Model file for the job. Use its own axes, mm. Face numbers are marked on the shaded views. Coordinates: 2 decimals unless noted, no trailing zeros. Order: outer loops, then holes, each group sorted by start corner. A loop starts at its lowest first (then second) coordinate and runs counter-clockwise, first axis right, second up. Notation, with made-up numbers: (36.25, 69) -> (86.25, 69) arc R15 ccw to (86.25, 76) -> close; hole circle Ø4 at (54, 70.25). An arc over 180 degrees is marked (long way). Return JSON: item names as keys, results as strings. Group by question number.
1) Pull direction X, two halves, no side cores. Call the marked faces 1, 2, 3 and 4: +X half, -X half, draft (parallel to the pull), parting line (faces both ways), or undercut.
2) Flat gauge pins, fed straight in: pin 1 (1 mm diameter, centred on y = -2.5, z = 3, fed in from +X); pin 2 (1 mm diameter, centred on x = 3.5, y = 1, fed in from -Z); pin 3 (2 mm diameter, centred on x = 0.5, z = -2, fed in from +Y). Where does each tip first touch, or does it go through?
3) Cut at D-D (x = 4.75). Write the cut outline in (y, z) (1 decimal), and give its area (3 significant figures).
4) Probe line 1 (Z direction, x = -0.75, y = 0) (3 decimals); line 2 (Y direction, x = -3.75, z = 1); line 3 (Z direction, x = 4.25, y = 1). List the from-to ranges inside material, lowest first.
5) Cut at C-C (x = -4.5). Write the cut outline in (y, z) (3 decimals), and give its area (3 significant figures).
Autodesk Inventor part; units mm, degrees
ref_plane "作業平面1" through (4.5, 0, 0) normal (1, 0, 0) x (0, 0, -1)
ref_plane "YZ Plane" through (0, 0, 0) normal (1, 0, 0) x (0, 1, 0)
ref_plane "XZ Plane" through (0, 0, 0) normal (0, 1, 0) x (-1, 0, 0)
sketch "スケッチ1" plane through (0, 0, 0) normal (1, 0, 0) x (0, 1, 0)
  circle A0 centre (0, 0) radius 3.635
  circle A1 centre (0, 0) radius 1.635
  circle A2 centre (0, 0) radius 2.635
  dimension "d0" = 3.27
  dimension "d1" = 2
  dimension "d7" = 1
extrude "押し出し1" add sketch "スケッチ1" along normal mid plane 11 contours A0 | A2
ref_plane "作業平面1" through (4.5, 0, 0) normal (1, 0, 0) x (0, 0, -1)
extrude "押し出し3" cut sketch "スケッチ1" against normal blind 1 from surface at 4.5 contours A0
chamfer "面取り3" distance 1 angle 45 1 edges at (5.5, -3.635, 0)
properties part number "spacer_Φ3.2_1"
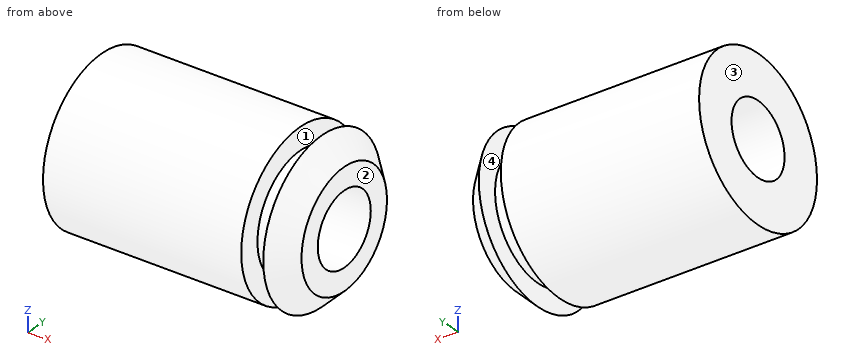
Answers below:
{
 "1": {"face 1": "undercut", "face 2": "+X half", "face 3": "-X half", "face 4": "undercut"},
 "2": {"pin 1": "stops at x = 4.73", "pin 2": "stops at z = -3.6", "pin 3": "stops at y = 3.49"},
 "3": {"outline": "circle Ø6.8 at (0, 0); hole circle Ø3.3 at (0, 0)", "area": "27.6 mm^2"},
 "4": {"line 1": "z = -3.635 to -1.635, 1.635 to 3.635", "line 2": "y = -3.49 to -1.29, 1.29 to 3.49", "line 3": "z = -2.44 to -1.29, 1.29 to 2.44"},
 "5": {"outline": "circle Ø7.27 at (0, 0); hole circle Ø3.27 at (0, 0)", "area": "33.1 mm^2"}
}
